Drawing for the job (mm, zero at the part's lowest x, y, z). A direction names the side the tool comes from. Give positions to 0.01 mm unless a question says otherwise; leave off trailing zeros. Loops run counter-clockwise (first coordinate to the right, second up) from the corner with the lowest first, then second, coordinate; pieces in that order, holes last. Notation, with made-up numbers: (23, 51) -> (30, 51) arc R20 cw to (30, 86) -> close; hole circle Ø4 at (14.25, 79). An arc over 180 degrees is marked (long way). Use CSV: the item, a comma, the result in double quotes. Start each with the question number.
(1) Cut at B-B on y = 39.5. Write the cut outline in (x, z).
(2) Cut at A-A on z = 123.5. Write the cut outline in (x, y).
(3) Flat gauge pins, fed straight in: pin 1 (4 mm diameter, centred on y = 27.5, z = 136, fed in from -X); pin 2 (6 mm diameter, centred on y = 23.5, z = 23.5, fed in from -X); pin 3 (1.5 mm diameter, centred on x = 249, y = 69, fed in from +Z). Where does each tip first touch, or does it go through?
(4) Drill centre lines: probe 1 along X at (y, z) = (10, 137.5); probe 2 along Z at (x, y) = (214.5, 78.5); probe 3 along X at (y, z) = (71, 139) (1 decimal). Where is each one in solid material? Low to high.
(5) 3-axis set-ups, long thin cutter, end or side, ignore diameter. For the marked faces 1, 2 and 3: which of +Z, -Z, +X, -X, +Y, -Y reach the whole face in a straight line?
(6) Cut at D-D on z = 54.5. Write the cut outline in (x, y) (3 decimals), then the cut area to 3 significant figures.
(7) Cut at C-C on x = 222. Write the cut outline in (y, z).
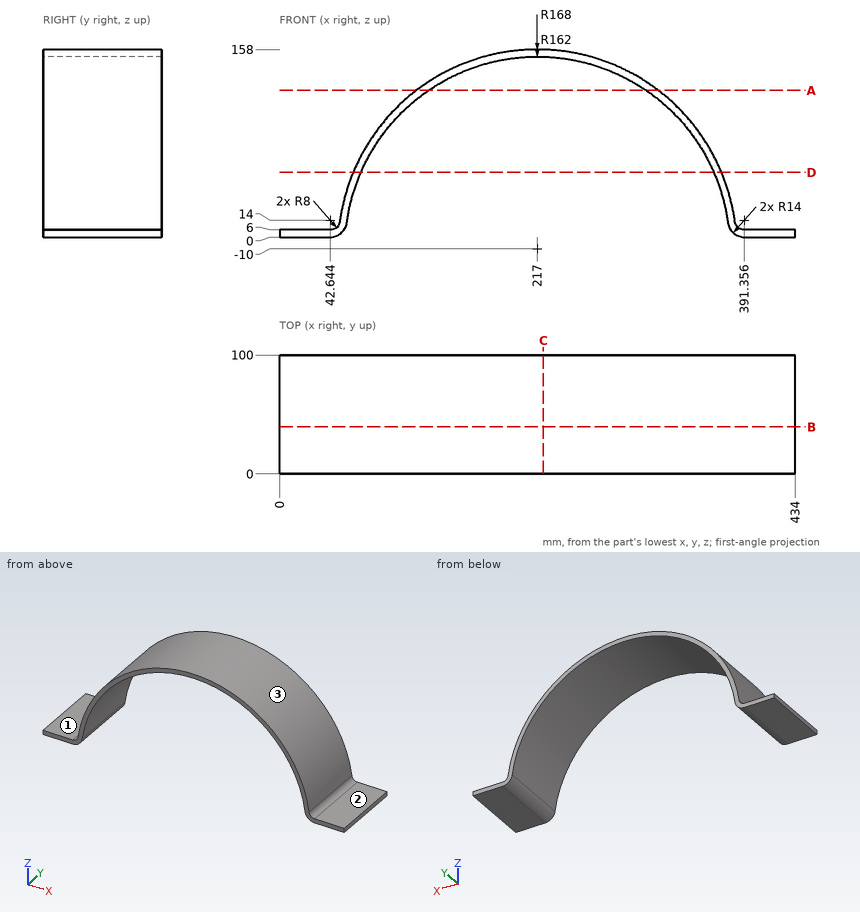
Check result:
1,outline,"(0, 0) -> (42.64, 0) arc R14 ccw to (56.51, 12.09) arc R162 cw to (377.49, 12.09) arc R14 ccw to (391.36, 0) -> (434, 0) -> (434, 6) -> (391.36, 6) arc R8 cw to (383.43, 12.91) arc R168 ccw to (50.57, 12.91) arc R8 cw to (42.64, 6) -> (0, 6) -> close"
2,outline,"(115.01, 0) -> (125.23, 0) -> (125.23, 100) -> (115.01, 100) -> close; (308.77, 0) -> (318.99, 0) -> (318.99, 100) -> (308.77, 100) -> close"
3,pin 1,"x = 130.47"
3,pin 2,"x = 51.79"
3,pin 3,"z = 155.07"
4,probe 1,"136.58 to 150.01, 283.99 to 297.42"
4,probe 2,"151.98 to 157.98"
4,probe 3,"139.4 to 153.4, 280.6 to 294.6"
5,face 1,"+Z, -X, +Y, -Y"
5,face 2,"+Z, +X, +Y, -Y"
5,face 3,"+Z, +Y, -Y"
6,outline,"(61.875, 0) -> (68.394, 0) -> (68.394, 100) -> (61.875, 100) -> close; (365.606, 0) -> (372.125, 0) -> (372.125, 100) -> (365.606, 100) -> close"
6,area,"1,300 mm²"
7,outline,"(0, 151.92) -> (100, 151.92) -> (100, 157.93) -> (0, 157.93) -> close"
